Source: CAD feature listing. Evaluate the final solid. Frame: model axes, mm. A direction names the side the tool comes from. Coordinates: 2 decimals unless noted, no trailing zeros. Order: outer loops, then holes, each group sorted by start corner. A loop starts at its lowest first (then second) coordinate and runs counter-clockwise, first axis right, second up. Notation, with made-up numbers: (-6.75, -12.5) - (35.25, -12.5) arc R14 ccw to (35.25, -8.5) - close; hole circle Ø9 at (-31.5, 40). An arc over 180 degrees is marked (long way). One line per question, with ' | ' between items. Start each with the question number.
(1) Section A-A (z = -0.9). Return the cut outline in (x, y), then the cut area to 3 significant figures.
(2) Contact query for flat-ended pins moving along their axis: P1, Ø2, axis at x = 8.5, z = -1.5, coming from the +Y side; P2, Ø2, axis at x = 2.5, z = -1.5, coming from the -Y side; P3, Ø0.6, axis at y = -21, z = -1.5, coming from the -X side. Output: stop coordinate, or through.
(3) Section B-B (x = -20). Return the cut outline in (y, z).
(4) Section C-C (y = -17). Return the cut outline in (x, z).
(5) Draft query along Y for faces 1 (the flat face through (0, -6, 0)), 2 (the flat face through (0, -10, -1)), 3 (the flat face through (0, 0, 1)). Return one class per face: +Y half, -Y half, draft (parallel to the pull), parting line (faces both ways), or undercut.
(6) Line query: line 1 along Y through (x, z) = (1.5, -0.6); line 2 along X through (y, z) = (-12, -1.2); line 3 along Z through (x, y) = (-21, -24). Output: solid intervals per line, ascending.
(7) Access query for faces 4 (the flat face through (-26.5, -20, -1)), 5 (the flat face through (25.5, -20, -1)), 6 (the flat face through (0, -31, -1)). Directions: +Z, -Z, +X, -X, +Y, -Y. A direction counts if a zero-diameter tool reaches every point of the face in a straight line with its end or side. Return the directions, or none.
Autodesk Inventor part; units mm, degrees
ref_plane "YZ Plane" through (0, 0, 0) normal (1, 0, 0) x (0, 1, 0)
ref_plane "XZ Plane" through (0, 0, 0) normal (0, 1, 0) x (-1, 0, 0)
ref_plane "XY Plane" through (0, 0, 0) normal (0, 0, 1) x (1, 0, 0)
sketch "Sketch1" plane through (0, 0, 0) normal (0, 0, 1) x (1, 0, 0)
  spline S0 degree 3 poles (-30, -5) (-30, -4.3586) (-29.8694, -3.6802) (-29.3471, -2.4395) (-28.9555, -1.8763) (-28.0866, -1.0236) (-27.5672, -0.665) (-27, -0.4174) knots 1.621626 1.621626 1.621626 1.621626 1.814042 1.814042 2.006457 2.006457 2.182648 2.182648 2.182648 2.182648
  line L0 (-25, 0) -> (25, 0)
  spline S1 degree 3 poles (27, -0.4174) (27.5672, -0.665) (28.0866, -1.0236) (28.9555, -1.8763) (29.3471, -2.4395) (29.8694, -3.6802) (30, -4.3586) (30, -5) knots -0.561022 -0.561022 -0.561022 -0.561022 -0.384831 -0.384831 -0.192415 -0.192415 0 0 0 0
  line L1 (30, -5) -> (30, -35)
  spline S2 degree 3 poles (30, -35) (30, -35.6414) (29.8694, -36.3198) (29.3471, -37.5605) (28.9555, -38.1237) (28.0866, -38.9764) (27.5672, -39.335) (27, -39.5826) knots 0 0 0 0 0.192415 0.192415 0.384831 0.384831 0.561022 0.561022 0.561022 0.561022
  line L2 (25, -40) -> (-25, -40)
  line L3 (-30, -35) -> (-30, -5)
  spline S3 degree 3 poles (-27, -39.5826) (-27.5672, -39.335) (-28.0866, -38.9764) (-28.9555, -38.1237) (-29.3471, -37.5605) (-29.8694, -36.3198) (-30, -35.6414) (-30, -35) knots 1.060605 1.060605 1.060605 1.060605 1.236796 1.236796 1.429211 1.429211 1.621626 1.621626 1.621626 1.621626
  arc A0 (-25, 0) -> (-27, -0.4174) centre (-25, -5) ccw
  arc A1 (27, -0.4174) -> (25, 0) centre (25, -5) ccw
  arc A2 (25, -40) -> (27, -39.5826) centre (25, -35) ccw
  arc A3 (-27, -39.5826) -> (-25, -40) centre (-25, -35) ccw
  point P0 (0, 0)
  dimension "d8" = 60
  dimension "d9" = 40
extrude "Extrusion1" add sketch "Sketch1" along normal blind 2.5
sketch "Sketch2" plane through (0, 0, 0) normal (0, 0, -1) x (-1, 0, 0)
  line L0 (-25.5, -10) -> (25.5, -10)
  line L1 (25.5, -10) -> (25.5, -30)
  line L2 (25.5, -30) -> (-25.5, -30)
  line L3 (-25.5, -30) -> (-25.5, -10)
  line L4 (-25.5, -10) -> (25.5, -30) construction
  line L5 (25.5, -10) -> (-25.5, -30) construction
  line L6 (-26.5, -9) -> (26.5, -9)
  line L7 (26.5, -9) -> (26.5, -31)
  line L8 (26.5, -31) -> (-26.5, -31)
  line L9 (-26.5, -31) -> (-26.5, -9)
  line L10 (-26.5, -9) -> (26.5, -31) construction
  line L11 (26.5, -9) -> (-26.5, -31) construction
  point P0 (0, 0)
  point P1 (0, -20)
  point P2 (0, -20)
  dimension "d2" = 51
  dimension "d3" = 20
  dimension "d4" = 53
  dimension "d5" = 22
extrude "Extrusion2" add sketch "Sketch2" along normal blind 2
properties part number "obudowa - budzik v3 plexi" material "Glass"
Response values:
1) outline: (-26.5, -31) - (26.5, -31) - (26.5, -9) - (-26.5, -9) - close; hole (-25.5, -30) - (25.5, -30) - (25.5, -10) - (-25.5, -10) - close | area: 146 mm²
2) P1: stops at y = -9 | P2: stops at y = -31 | P3: stops at x = -26.5
3) outline: (-40, 0) - (-31, 0) - (-31, -2) - (-30, -2) - (-30, 0) - (-10, 0) - (-10, -2) - (-9, -2) - (-9, 0) - (0, 0) - (0, 2.5) - (-40, 2.5) - close
4) outline: (-30, 0) - (-26.5, 0) - (-26.5, -2) - (-25.5, -2) - (-25.5, 0) - (25.5, 0) - (25.5, -2) - (26.5, -2) - (26.5, 0) - (30, 0) - (30, 2.5) - (-30, 2.5) - close
5) face 1: draft | face 2: undercut | face 3: +Y half
6) line 1: y = -31 to -30, -10 to -9 | line 2: x = -26.5 to -25.5, 25.5 to 26.5 | line 3: z = 0 to 2.5
7) face 4: -Z, -X, +Y, -Y | face 5: -Z | face 6: -Z, +X, -X, -Y
